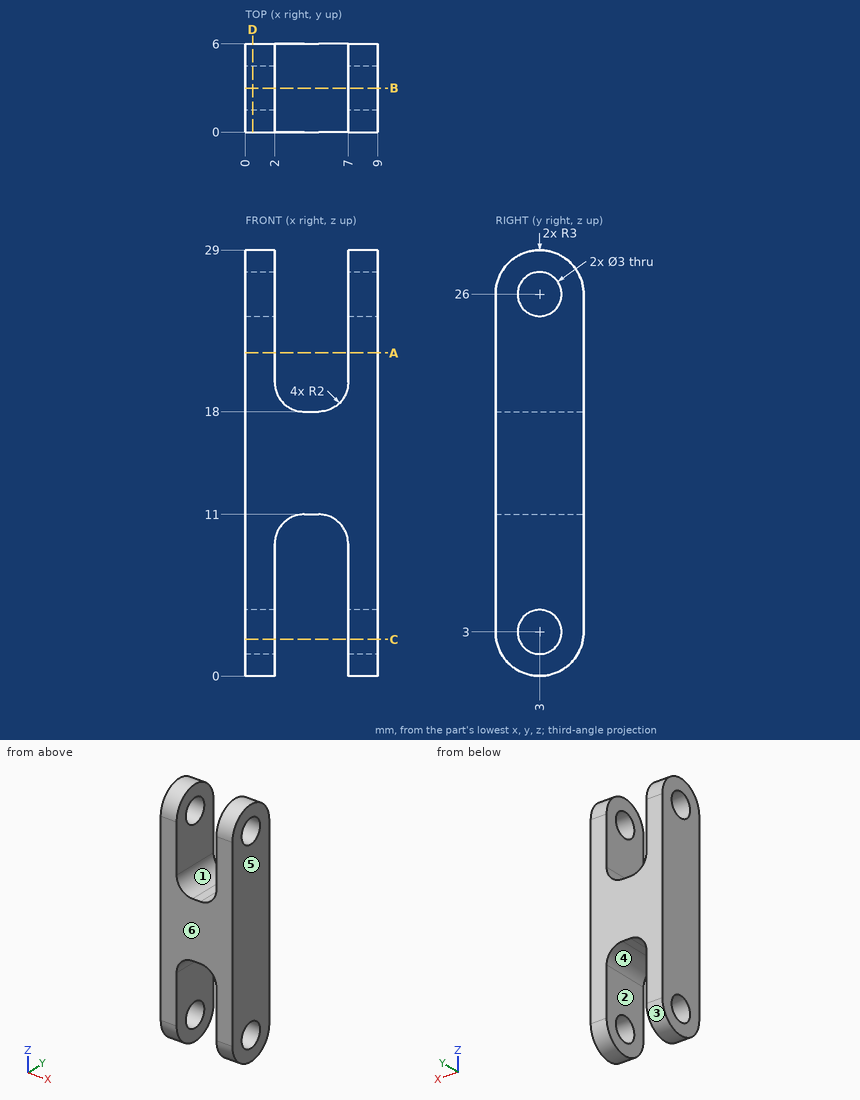
Can you work these out from the drawing? Everything is in mm from the part's minimum corner. A direction names the side the tool comes from. Round coordinates to 2 decimals unless told otherwise and drop trailing zeros. Loops run counter-clockwise (first coordinate to the right, second up) from the corner with the lowest first, then second, coordinate; pieces in that order, holes last.
1. If we section it at A-A on z = 22: Write out the boundary of the cut face in (x, y), plus the area to 3 significant figures.
Answer list:
outline: (0, 0) - (2, 0) - (2, 6) - (0, 6) - close; (7, 0) - (9, 0) - (9, 6) - (7, 6) - close
area: 24.0 mm2
2. For P1, Ø2.5, axis at y = 3, z = 3, coming from the +X side; P2, Ø0.8, axis at x = 4.5, y = 3.5, coming from the -Z side, each with a flat end and sliding along its axis, tell me the tip position at first contact or that it passes through.
Answer list:
P1: passes through
P2: stops at z = 11
3. If we section it at C-C on z = 2.5: Write out the boundary of the cut face in (x, y), plus the area to 3 significant figures.
Answer list:
outline: (0, 0.04) - (2, 0.04) - (2, 1.59) - (0, 1.59) - close; (0, 4.41) - (2, 4.41) - (2, 5.96) - (0, 5.96) - close; (7, 0.04) - (9, 0.04) - (9, 1.59) - (7, 1.59) - close; (7, 4.41) - (9, 4.41) - (9, 5.96) - (7, 5.96) - close
area: 12.4 mm2
4. If I drill on line 1 along Y through (x, z) = (7.45, 3); line 2 along X through (y, z) = (5, 6.5); line 3 along Z through (x, y) = (7.5, 2.3), over which ranges is the centre line in solid material (lowest first)?
Answer list:
line 1: y = 0 to 1.5, 4.5 to 6
line 2: x = 0 to 2, 7 to 9
line 3: z = 0.08 to 1.67, 4.33 to 24.67, 27.33 to 28.92
5. If we section it at B-B on y = 3: Count the separate pieces of the cut face and the enclosed holes in it, plus the area to 3 significant figures.
Answer list:
separate pieces: 5
enclosed holes: 0
area: 130 mm2
6. Which directions (+Z, -Z, +X, -X, +Y, -Y) give clear straight access to the entire face, cutting with the end or side of a thin tool? Please do the marked faces 1, 2 and 3.
Answer list:
face 1: +Z, +Y, -Y
face 2: -Z, +Y, -Y
face 3: -Z, +X, -X
7. If we section it at D-D on x = 0.5: Write out the boundary of the cut face in (y, z), plus the area to 3 significant figures.
Answer list:
outline: (0, 3) arc R3 ccw to (6, 3) - (6, 26) arc R3 ccw to (0, 26) - close; hole circle Ø3 at (3, 3); hole circle Ø3 at (3, 26)
area: 152 mm2
8. We'd pull the mould along X, two halves only. Please class the marked faces 4, 5 and 6: +X half, -X half, draft (parallel to the pull), parting line (faces both ways), or undercut.
Answer list:
face 4: undercut
face 5: +X half
face 6: draft
